Autodesk Inventor part; units mm, degrees
ref_plane "YZ Plane" through (0, 0, 0) normal (1, 0, 0) x (0, 1, 0)
ref_plane "XZ Plane" through (0, 0, 0) normal (0, 1, 0) x (-1, 0, 0)
ref_plane "XY Plane" through (0, 0, 0) normal (0, 0, 1) x (1, 0, 0)
sketch "Sketch1" plane through (0, 0, 0) normal (1, 0, 0) x (0, 1, 0)
  line L0 (0, 0) -> (25.4, 0)
  line L1 (25.4, 0) -> (25.4, -15.875)
  line L2 (25.4, -15.875) -> (0, -15.875)
  line L3 (0, -15.875) -> (0, 0)
  dimension "d0" = 25.4
  dimension "d1" = 15.875
extrude "Extrusion1" add sketch "Sketch1" along normal blind 117.475
chamfer "Chamfer1" distance 0.762 angle 45 11 edges at (117.475, 12.7, 0) (117.475, 12.7, -15.875) (117.475, 0, -7.9375) (58.7375, 0, 0) (58.7375, 25.4, 0) (58.7375, 25.4, -15.875) (0, 12.7, 0) (0, 25.4, -7.9375) (0, 12.7, -15.875) (0, 0, -7.9375) (58.7375, 0, -15.875)
sketch "Sketch2" plane through (0.762, 25.4, -15.113) normal (0, 1, 0) x (1, 0, 0)
  line L0 (0, -15.113) -> (115.951, -15.113)
  line L1 (0, -15.113) -> (7.9375, -15.113)
  line L2 (7.9375, -15.113) -> (7.9375, -7.1755)
  point P0 (-0.762, -15.113)
  dimension "d7" = 7.9375
  dimension "d8" = 7.9375
hole "Hole1" at (8.6995, 25.4, -7.9375) direction (0, -1, 0) diameter 7.9375 end through all countersink diameter 9.525 countersink angle 82
sketch "Sketch3" plane through (0.762, 25.4, -15.113) normal (0, 1, 0) x (1, 0, 0)
  line L0 (116.713, 0) -> (116.713, -14.351)
  line L1 (116.713, -7.1755) -> (45.2755, -7.1755)
  point P0 (-0.762, -15.113)
  dimension "d16" = 71.4375
hole "Hole2" at (46.0375, 25.4, -7.9375) direction (0, -1, 0) diameter 6.35 end through all countersink diameter 7.9375 countersink angle 82
sketch "Sketch4" plane through (0.762, 25.4, -15.113) normal (0, 1, 0) x (1, 0, 0)
  line L0 (116.713, 0) -> (116.713, -14.351)
  line L1 (116.713, -7.1755) -> (62.738, -7.1755)
  point P0 (-0.762, -15.113)
  dimension "d24" = 53.975
hole "Hole3" at (63.5, 25.4, -7.9375) direction (0, -1, 0) diameter 11.1125 end through all countersink diameter 12.7 countersink angle 82
sketch "Sketch5" plane through (0.762, 25.4, -15.113) normal (0, 1, 0) x (1, 0, 0)
  line L0 (116.713, 0) -> (116.713, -14.351)
  line L1 (116.713, -7.1755) -> (108.7755, -7.1755)
  point P0 (-0.762, -15.113)
  dimension "d32" = 7.9375
hole "Hole4" at (109.5375, 25.4, -7.9375) direction (0, -1, 0) diameter 7.9375 end through all countersink diameter 9.525 countersink angle 82
sketch "Sketch6" plane through (0.762, 0.762, 0) normal (0, 0, 1) x (1, 0, 0)
  line L0 (111.9534, -0.762) -> (111.9534, 4.8006) construction
  line L1 (117.1134, 4.8006) -> (90.1259, 4.8006) construction
  point P0 (-0.762, -0.762)
  dimension "d40" = 5.5626
  dimension "d41" = 26.9875
hole "Hole5" at (90.8879, 5.5626, 0) direction (0, 0, -1) diameter 4.7625 end through all countersink diameter 6.35 countersink angle 82
sketch "Sketch7" plane through (0.762, 0.762, 0) normal (0, 0, 1) x (1, 0, 0)
  line L0 (114.57, -0.762) -> (114.57, 16.7005)
  line L1 (116.5466, 16.7005) -> (75.2716, 16.7005)
  point P0 (-0.762, -0.762)
  dimension "d49" = 17.4625
  dimension "d50" = 41.275
hole "Hole6" at (76.0336, 17.4625, 0) direction (0, 0, -1) diameter 6.35 end through all countersink diameter 7.9375 countersink angle 82
chamfer "Chamfer2" distance 0.762 angle 45 1 edges at (117.475, 25.4, -7.9375)
properties part number "holes1"
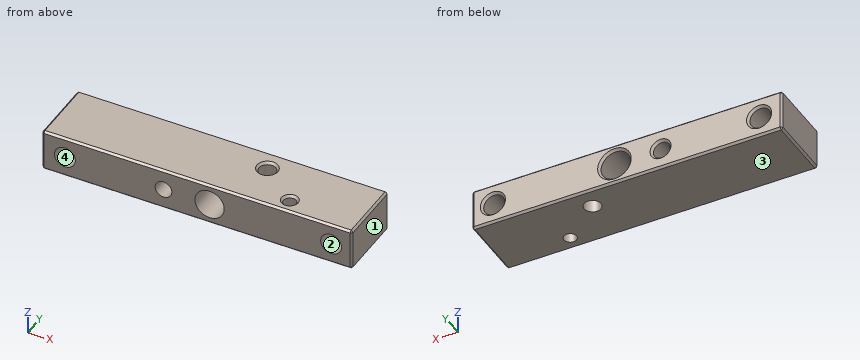
Geometry: final body of the model. Coordinates: model frame, mm. Face numbers are marked on the shaded views. Coordinates: 2 decimals unless noted, no trailing zeros. Order: outer loops, then holes, each group sorted by start corner. A loop starts at its lowest first (then second) coordinate and runs counter-clockwise, first axis right, second up. Notation, with made-up numbers: (78, -12.5) -> (82, -12.5) arc R20 cw to (82, -8.5) -> close; hole circle Ø3 at (3.5, -4.75). An arc over 180 degrees is marked (long way). Write each question's results on one line, items separated by ' | '. Start each with the question number.
1) Material intervals for line 1 along X through (y, z) = (16, -7) (1 decimal); line 2 along X through (y, z) = (16.25, -12.75) (3 decimals); line 3 along Y through (x, z) = (76, -4.25), sorted ascending.
2) First-contact query: pin 1 (9 mm diameter, centred on x = 109.54, z = -7.94, fed in from +Y). Flat tip, straight axial feed; report the tip coordinate or a pass-through.
3) Cut plane A-A, the plane x = 63.5. Output: boundary loops of the cut face in (y, z) (1 decimal), and give its area (3 significant figures).
4) Mould query, pull axis X, two halves, no side actions, for the marked faces 1, 2, 3 and 4. Classes: released by +X, released by -X, zero draft, split by the parting line, or undercut.
5) Cut plane B-B, the plane z = -8.75. State how many separate pieces and enclosed holes the cut face has, and give its area (3 significant figures).
Checks:
1) line 1: 0 to 4.8, 12.6 to 43, 49.1 to 58, 69 to 73.2, 78.9 to 105.7, 113.4 to 117.5 | line 2: 0 to 60.723, 66.277 to 73.099, 78.968 to 117.475 | line 3: 0 to 14.29, 20.64 to 25.4
2) pin 1: y = 25.1
3) outline: (0, -15.1) -> (0.8, -15.9) -> (24.6, -15.9) -> (25.4, -15.1) -> (25.4, -14.3) -> (24.5, -13.5) -> (0, -13.5) -> close; (0, -2.4) -> (24.5, -2.4) -> (25.4, -1.6) -> (25.4, -0.8) -> (24.6, 0) -> (0.8, 0) -> (0, -0.8) -> close | area: 119 mm^2
4) face 1: released by +X | face 2: undercut | face 3: zero draft | face 4: undercut
5) separate pieces: 5 | enclosed holes: 2 | area: 2,100 mm^2
